```python
from build123d import *

# Parameters (mm, degrees)
SKETCH_W         = 150
SKETCH_H         = 150
PAD_DEPTH        = 30
SKETCH001_R      = 3
PAD001_DEPTH     = 1
SKETCH002_R      = 1.75
POCKET_DEPTH     = 20
SKETCH003_R      = 5
PAD002_DEPTH     = 0.5
SKETCH004_W      = 20
SKETCH004_H      = 10
POCKET001_DEPTH  = 1
SKETCH005_W      = 16
SKETCH005_H      = 6
REVOLUTION_ANGLE = 20
CHAMFER_SIZE     = 4


with BuildPart() as part:
    # Sketch → Pad (new body, symmetric)
    with BuildSketch(Plane.XY):
        Rectangle(SKETCH_W, SKETCH_H)
    extrude(amount=PAD_DEPTH, both=True)

    # Sketch001 (on Face6 of Pad) → Pad001 (join)
    with BuildSketch(Plane.XY.offset(30)):
        with Locations((-30, 30)):
            Circle(SKETCH001_R)
        with Locations((0, 30)):
            Circle(SKETCH001_R)
        with Locations((30, 30)):
            Circle(SKETCH001_R)
        with Locations((-30, 0)):
            Circle(SKETCH001_R)
        Circle(SKETCH001_R)
        with Locations((30, 0)):
            Circle(SKETCH001_R)
        with Locations((-30, -30)):
            Circle(SKETCH001_R)
        with Locations((0, -30)):
            Circle(SKETCH001_R)
        with Locations((30, -30)):
            Circle(SKETCH001_R)
    extrude(amount=PAD001_DEPTH)

    # Sketch002 (on Face5 of Pad001) → Pocket (cut)
    with BuildSketch(Plane.XY.offset(31)):
        with Locations((-30, 30)):
            Circle(SKETCH002_R)
        with Locations((0, 30)):
            Circle(SKETCH002_R)
        with Locations((30, 30)):
            Circle(SKETCH002_R)
        with Locations((-30, 0)):
            Circle(SKETCH002_R)
        Circle(SKETCH002_R)
        with Locations((30, 0)):
            Circle(SKETCH002_R)
        with Locations((-30, -30)):
            Circle(SKETCH002_R)
        with Locations((0, -30)):
            Circle(SKETCH002_R)
        with Locations((30, -30)):
            Circle(SKETCH002_R)
    extrude(amount=-POCKET_DEPTH, mode=Mode.SUBTRACT)

    # Sketch003 (on Face5 of Pocket) → Pad002 (join)
    with BuildSketch(Plane.XY.offset(30)):
        with Locations((-30, 30)):
            Circle(SKETCH003_R)
        with Locations((0, 30)):
            Circle(SKETCH003_R)
        with Locations((30, 30)):
            Circle(SKETCH003_R)
        with Locations((-30, 0)):
            Circle(SKETCH003_R)
        Circle(SKETCH003_R)
        with Locations((30, 0)):
            Circle(SKETCH003_R)
        with Locations((-30, -30)):
            Circle(SKETCH003_R)
        with Locations((0, -30)):
            Circle(SKETCH003_R)
        with Locations((30, -30)):
            Circle(SKETCH003_R)
    extrude(amount=PAD002_DEPTH)

    # Sketch004 (on Face1 of Pad002) → Pocket001 (cut)
    with BuildSketch(Plane.XZ.offset(75)):
        with Locations((-40, -20)):
            Rectangle(SKETCH004_W, SKETCH004_H)
    extrude(amount=-POCKET001_DEPTH, mode=Mode.SUBTRACT)

    # Sketch005 (on Face20 of Pocket001) → Revolution (revolve)
    with BuildSketch(Plane.XZ.offset(74)):
        with Locations((-40, -20)):
            Rectangle(SKETCH005_W, SKETCH005_H)
    revolve(axis=Axis((-32, -74, -23), (0, 0, 1)), revolution_arc=REVOLUTION_ANGLE)

    # Chamfer
    chamfer_edges = [part.edges().sort_by_distance(p)[0] for p in [
        (0, 75, 30),
        (75, 0, 30),
        (0, -75, 30),
        (-75, 0, 30),
    ]]
    chamfer(chamfer_edges, length=CHAMFER_SIZE)


solid = part.part
```
Input: part model. Units: mm. Frame: model coordinates. A direction names the side the tool comes from. Give positions to 0.01 mm unless a question says otherwise; leave off trailing zeros. Loops run counter-clockwise (first coordinate to the right, second up) from the corner with the lowest first, then second, coordinate; pieces in that order, holes last. Notation, with made-up numbers: (54, 87) -> (65, 87) arc R7 cw to (65, 97) -> close; hole circle Ø8 at (-17.5, 79.5). An arc over 180 degrees is marked (long way). Use a Markdown table: item, result.
Q1. Ray query, probe 1 along Y at (x, z) = (30.5, 21); probe 2 along Y at (x, z) = (8, -23); probe 3 along Z at (x, y) = (39, 36). Return the intervals inside material, ascending. Write a range as from..to.
Entries:
| item | result |
|---|---|
| probe 1 | y = -75..-31.68, -28.32..-1.68, 1.68..28.32, 31.68..75 |
| probe 2 | y = -75..75 |
| probe 3 | z = -30..30 |
Q2. First-contact query: P1, Ø5, axis at x = 20, y = -38.5, coming from the +Z side; P2, Ø4, axis at x = -1, y = 0.5, coming from the +Z side; P3, Ø2, axis at x = 30, y = -30, coming from the +Z side; P4, Ø2.5, axis at x = -44, y = -77.5, coming from the +Z side. Flat tips, straight axial feed; report the tip coordinate or a pass-through.
Entries:
| item | result |
|---|---|
| P1 | stops at z = 30 |
| P2 | stops at z = 31 |
| P3 | stops at z = 30.5 |
| P4 | stops at z = -17 |
Q3. Section query D-D, the plane z = -10. Return the cut outline in (x, y).
Entries:
| item | result |
|---|---|
| outline | (-75, -75) -> (75, -75) -> (75, 75) -> (-75, 75) -> close |
Q4. Section query B-B, the plane x = 20. Return the cut outline in (y, z).
Entries:
| item | result |
|---|---|
| outline | (-75, -30) -> (75, -30) -> (75, 26) -> (71, 30) -> (-71, 30) -> (-75, 26) -> close |
Q5. Pull-direction query (X, two-part tool) for faces 5 (the flat face through (0, -32, 31)), 6 (the cylindrical face through (-31.75, 30.08, 30.75)); classes: pulls with the +X half, pulls with the -X half, needs draft (parallel to the pull), parting line crosses it, or undercut.
Entries:
| item | result |
|---|---|
| face 5 | needs draft |
| face 6 | undercut |
Q6. Access query for faces 1 (the flat face through (0, 28, 31)), 2 (the cylindrical face through (-47.764, -76.74, -19.958)), 3 (the flat face through (-0.1, 26.7, 30.5)), 4 (the flat face through (-30, 30, 11)). Directions: +Z, -Z, +X, -X, +Y, -Y. A direction counts if a zero-diameter tool reaches every point of the face in a straight line with its end or side. Return the directions, or none.
Entries:
| item | result |
|---|---|
| face 1 | +Z, +X, -X, +Y, -Y |
| face 2 | -Y |
| face 3 | +Z |
| face 4 | none |
Q7. Section query A-A, the plane z = 17. State how many separate pieces and enclosed holes the cut face has, plus the area to 3 significant figures.
Entries:
| item | result |
|---|---|
| separate pieces | 1 |
| enclosed holes | 9 |
| area | 22,400 mm² |
